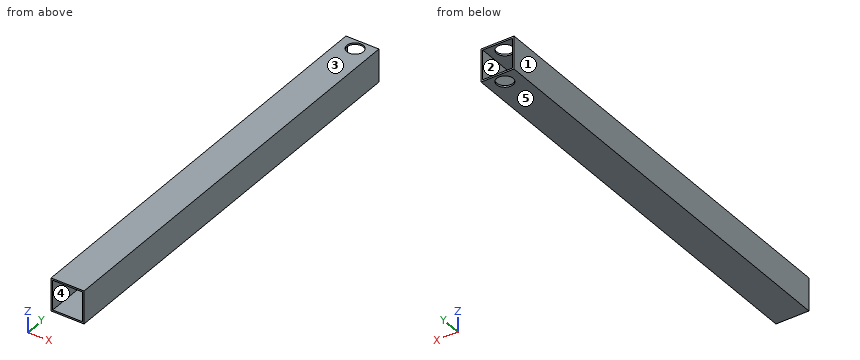
Autodesk Inventor part; units mm, degrees
ref_plane "YZ Plane" through (0, 0, 0) normal (1, 0, 0) x (0, 1, 0)
ref_plane "XZ Plane" through (0, 0, 0) normal (0, 1, 0) x (-1, 0, 0)
ref_plane "XY Plane" through (0, 0, 0) normal (0, 0, 1) x (1, 0, 0)
sketch "Sketch1" plane through (0, 0, 0) normal (0, 1, 0) x (-1, 0, 0)
  line L0 (-12.7, -12.7) -> (12.7, -12.7)
  line L1 (12.7, -12.7) -> (12.7, 12.7)
  line L2 (12.7, 12.7) -> (-12.7, 12.7)
  line L3 (-12.7, 12.7) -> (-12.7, -12.7)
  line L4 (-12.7, -12.7) -> (12.7, 12.7) construction
  line L5 (12.7, -12.7) -> (-12.7, 12.7) construction
  line L6 (-11.43, -11.43) -> (11.43, -11.43)
  line L7 (11.43, -11.43) -> (11.43, 11.43)
  line L8 (11.43, 11.43) -> (-11.43, 11.43)
  line L9 (-11.43, 11.43) -> (-11.43, -11.43)
  line L10 (-11.43, -11.43) -> (11.43, 11.43) construction
  line L11 (11.43, -11.43) -> (-11.43, 11.43) construction
  point P0 (0, 0)
  dimension "d0" = 25.4
  dimension "d1" = 25.4
  dimension "d2" = 22.86
  dimension "d3" = 22.86
extrude "Extrusion1" add sketch "Sketch1" along normal blind 327.3044
sketch "Sketch2" plane through (0, 327.3044, 0) normal (0, 1, 0) x (1, 0, 0)
  line L0 (11.43, 11.43) -> (11.43, -11.43)
  line L1 (11.43, -11.43) -> (-11.43, -11.43)
  line L2 (-11.43, -11.43) -> (-11.43, 11.43)
  line L3 (-11.43, 11.43) -> (11.43, 11.43)
  line L4 (12.7, 12.7) -> (-12.7, 12.7)
  line L5 (-12.7, 12.7) -> (-12.7, -12.7)
  line L6 (-12.7, -12.7) -> (12.7, -12.7)
  line L7 (12.7, -12.7) -> (12.7, 12.7)
  point P0 (0, 0)
extrude "Extrusion2" add sketch "Sketch2" against normal blind 327.3044
sketch "Sketch5" plane through (12.7, 0, -12.7) normal (0, 0, -1) x (-1, 0, 0)
  circle A0 centre (12.7, 319.1401) radius 6.35
  line L0 (106.09, 453.881) -> (-174.2251, -6.5402) construction
  line L1 (78.7715, 457.8537) -> (-195.9205, 6.6684) construction
  line L2 (-0.7099, 327.3044) -> (20.9855, 314.0957) construction
  point P0 (12.7, 0)
  dimension "d12" = 12.7
extrude "Extrusion4" cut sketch "Sketch5" against normal blind 59.9694
equation "\"BendRadius\" = Thickness"
equation "\"BendReliefWidth\" = Thickness"
equation "\"BendReliefDepth\" = 0.5 * Thickness"
equation "\"CornerReliefSize\" = 4 * Thickness"
equation "\"MinimumRemnant\" = 2 * Thickness"
equation "\"TransitionRadius\" = BendRadius"
equation "\"JacobiRadiusSize\" = BendRadius"
equation "\"GapSize\" = Thickness"
properties part number "Convery frame2" material "Aluminum 6061"
Build history of the part. All positions in model axes, mm. Face numbers are marked on the shaded views. A direction names the side the tool comes from. Round coordinates to 2 decimals unless told otherwise and drop trailing zeros. Write each loop counter-clockwise with the first axis right and the second up, starting at its lowest first coordinate (ties: lowest second). Pieces come first, ordered by that corner, then holes. Notation, with made-up numbers: (39, -38.5) - (48, -38.5) arc R15 ccw to (48, -25.5) - close; hole circle Ø6 at (7.25, -17). An arc over 180 degrees is marked (long way). One line per question, with ' | ' between items.
1. Band-saw the part on A-A, the plane x = 0. Write the cut outline in (y, z), and give its area (3 significant figures).
Results are:
outline: (0, -12.7) - (312.79, -12.7) - (312.79, -11.43) - (0, -11.43) - close; (0, 11.43) - (312.79, 11.43) - (312.79, 12.7) - (0, 12.7) - close; (325.49, -12.7) - (327.3, -12.7) - (327.3, -11.43) - (325.49, -11.43) - close; (325.49, 11.43) - (327.3, 11.43) - (327.3, 12.7) - (325.49, 12.7) - close | area: 799 mm^2
2. Mould opens along Z. For the marked faces 3, 4 and 5 say: released by +Z, released by -Z, zero draft, split by the parting line, or undercut.
Results are:
face 3: released by +Z | face 4: undercut | face 5: released by -Z
3. Band-saw the part on B-B, the plane y = 191. Write the cut outline in (x, z).
Results are:
outline: (-12.7, -12.7) - (12.7, -12.7) - (12.7, 12.7) - (-12.7, 12.7) - close; hole (-11.43, -11.43) - (11.43, -11.43) - (11.43, 11.43) - (-11.43, 11.43) - close
4. Band-saw the part on C-C, the plane z = -4.5. Write the cut outline in (x, y), and give its area (3 significant figures).
Results are:
outline: (-12.7, 0) - (-11.43, 0) - (-11.43, 327.3) - (-12.7, 327.3) - close; (11.43, 0) - (12.7, 0) - (12.7, 327.3) - (11.43, 327.3) - close | area: 831 mm^2
5. Drill centre lines: line 1 along X through (y, z) = (217, 0); line 2 along Y through (x, z) = (0, -11.9). Where is each one in solid material? Low to high. Write a range as from..to.
Results are:
line 1: -12.7..-11.43, 11.43..12.7 | line 2: 0..312.79, 325.49..327.3
6. Tool access for the marked faces 1 and 2: list every direction of +Z, -Z, +X, -X, +Y, -Y with a clear straight run to the whole face (end or side of a thin tool).
Results are:
face 1: +Z, -Z, -X, +Y, -Y | face 2: +Y, -Y
